Build history of the part. All positions in model axes, mm. Round coordinates to 2 decimals unless told otherwise and drop trailing zeros. Loops run counter-clockwise (first coordinate to the right, second up) from the corner with the lowest first, then second, coordinate; pieces in that order, holes last. Notation, with made-up numbers: (-35, -28) - (-21, -28) arc R25 cw to (-21, -13) - close; hole circle Ø2 at (26.25, 63). An arc over 180 degrees is marked (long way). Put each result on its own line as item: value. Start each with the question number.
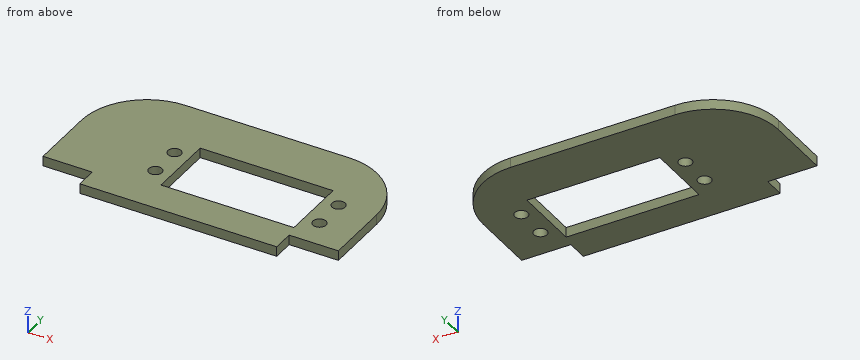
from build123d import *

# Parameters (mm, degrees)
SALIENTE_EXTRUIR1_DEPTH = 3
CORTAR_EXTRUIR1_REACH   = 5
CROQUIS2_W              = 40.5
CROQUIS2_H              = 20.5
REDONDEO1_R             = 20
CORTAR_EXTRUIR2_REACH   = 5
CROQUIS3_R              = 2


with BuildPart() as part:
    # Croquis1 → Saliente-Extruir1 (new body)
    with BuildSketch(Plane.XY):
        Polygon((-45, -20), (-30, -20), (-30, -26.5), (30, -26.5), (30, -20), (45, -20), (45, 20), (-45, 20), align=None)
    extrude(amount=SALIENTE_EXTRUIR1_DEPTH)

    # Croquis2 → Cortar-Extruir1 (cut, up to next)
    with BuildSketch(Plane.XY.offset(3), mode=Mode.PRIVATE) as cortar_extruir1_sk1:
        with Locations((9, -6)):
            Rectangle(CROQUIS2_W, CROQUIS2_H)
    cortar_extruir1_tool1 = extrude(cortar_extruir1_sk1.sketch, amount=-CORTAR_EXTRUIR1_REACH, mode=Mode.PRIVATE) & part.part
    add(cortar_extruir1_tool1.solids().sort_by_distance((9, -6, 3))[0], mode=Mode.SUBTRACT)

    # Redondeo1
    redondeo1_edges = [part.edges().sort_by_distance(p)[0] for p in [
        (-45, 20, 1.5),
        (45, 20, 1.5),
    ]]
    fillet(redondeo1_edges, radius=REDONDEO1_R)

    # Croquis3 → Cortar-Extruir2 (cut, up to next)
    with BuildSketch(Plane.XY.offset(3), mode=Mode.PRIVATE) as cortar_extruir2_sk1:
        with Locations((34, -1)):
            Circle(CROQUIS3_R)
    cortar_extruir2_tool1 = extrude(cortar_extruir2_sk1.sketch, amount=-CORTAR_EXTRUIR2_REACH, mode=Mode.PRIVATE) & part.part
    add(cortar_extruir2_tool1.solids().sort_by_distance((34, -1, 3))[0], mode=Mode.SUBTRACT)
    # Croquis3 → Cortar-Extruir2 (cut, up to next)
    with BuildSketch(Plane.XY.offset(3), mode=Mode.PRIVATE) as cortar_extruir2_sk2:
        with Locations((-16, -1)):
            Circle(CROQUIS3_R)
    cortar_extruir2_tool2 = extrude(cortar_extruir2_sk2.sketch, amount=-CORTAR_EXTRUIR2_REACH, mode=Mode.PRIVATE) & part.part
    add(cortar_extruir2_tool2.solids().sort_by_distance((-16, -1, 3))[0], mode=Mode.SUBTRACT)
    # Croquis3 → Cortar-Extruir2 (cut, up to next)
    with BuildSketch(Plane.XY.offset(3), mode=Mode.PRIVATE) as cortar_extruir2_sk3:
        with Locations((34, -11)):
            Circle(CROQUIS3_R)
    cortar_extruir2_tool3 = extrude(cortar_extruir2_sk3.sketch, amount=-CORTAR_EXTRUIR2_REACH, mode=Mode.PRIVATE) & part.part
    add(cortar_extruir2_tool3.solids().sort_by_distance((34, -11, 3))[0], mode=Mode.SUBTRACT)
    # Croquis3 → Cortar-Extruir2 (cut, up to next)
    with BuildSketch(Plane.XY.offset(3), mode=Mode.PRIVATE) as cortar_extruir2_sk4:
        with Locations((-16, -11)):
            Circle(CROQUIS3_R)
    cortar_extruir2_tool4 = extrude(cortar_extruir2_sk4.sketch, amount=-CORTAR_EXTRUIR2_REACH, mode=Mode.PRIVATE) & part.part
    add(cortar_extruir2_tool4.solids().sort_by_distance((-16, -11, 3))[0], mode=Mode.SUBTRACT)


solid = part.part
Item 1: Drop flat-ended pins along their axis: pin 1 Ø1.5 at (x, z) = (-40.5, 2) entering from -Y; pin 2 Ø1.5 at (y, z) = (-24.5, 2) entering from +X. Give the stop position or say it passes through.
Item 2: Drill centre lines: probe 1 along Y at (x, z) = (-16, 0.65); probe 2 along X at (y, z) = (-7, 2.5); probe 3 along Y at (x, z) = (-6.5, 2). Where is each one in solid material? Low to high. Write a range as [from, to].
Item 3: Slice it at A-A (y = -11). Give the cut face in (x, z), plus the area to 4 significant figures.
Item 4: Slice it at B-B (x = -16). Give the cut face in (y, z).
Item 5: Slice it at D-D (x = -5.5). Give the cut face in (y, z).
Item 6: Slice it at C-C (z = 1.55). Give the cut face in (x, y).
Computed values:
1. pin 1: stops at y = -20
1. pin 2: stops at x = 30
2. probe 1: y = [-26.5, -13], [-9, -3], [1, 20]
2. probe 2: x = [-45, -11.25], [29.25, 45]
2. probe 3: y = [-26.5, -16.25], [4.25, 20]
3. outline: (-45, 0) - (-18, 0) - (-18, 3) - (-45, 3) - close; (-14, 0) - (-11.25, 0) - (-11.25, 3) - (-14, 3) - close; (29.25, 0) - (32, 0) - (32, 3) - (29.25, 3) - close; (36, 0) - (45, 0) - (45, 3) - (36, 3) - close
3. area: 124.5 mm^2
4. outline: (-26.5, 0) - (-13, 0) - (-13, 3) - (-26.5, 3) - close; (-9, 0) - (-3, 0) - (-3, 3) - (-9, 3) - close; (1, 0) - (20, 0) - (20, 3) - (1, 3) - close
5. outline: (-26.5, 0) - (-16.25, 0) - (-16.25, 3) - (-26.5, 3) - close; (4.25, 0) - (20, 0) - (20, 3) - (4.25, 3) - close
6. outline: (-45, -20) - (-30, -20) - (-30, -26.5) - (30, -26.5) - (30, -20) - (45, -20) - (45, 0) arc R20 ccw to (25, 20) - (-25, 20) arc R20 ccw to (-45, 0) - close; hole circle Ø4 at (-16, -11); hole circle Ø4 at (-16, -1); hole (-11.25, -16.25) - (29.25, -16.25) - (29.25, 4.25) - (-11.25, 4.25) - close; hole circle Ø4 at (34, -11); hole circle Ø4 at (34, -1)
